Can you work these out from the model? Positions are in its coordinate system, mm. A direction names the side the tool comes from. Give positions to 0.01 mm unless a question says otherwise; leave off trailing zeros. Write each loop counter-clockwise with the first axis right and the second up, starting at its lowest first coordinate (ties: lowest second). Pieces come first, ordered by that corner, then holes.
from build123d import *

# Parameters (mm, degrees)
F1_DEPTH = 317.5
F4_DEPTH = 19.05
F5_DEPTH = 19.05


# Not quite as in the source:
# - a feature names something its author has since deleted; it is built from what else it names


with BuildPart() as f1:
    # F0 (on Front) → F1 (new body)
    with BuildSketch(Plane.XZ):
        with BuildLine():
            Line((152.4, 0), (0, 0))
            Line((0, 0), (0, -51.6636))
            Line((0, -51.6636), (8.7122, -51.6636))
            Line((8.7122, -51.6636), (8.7122, -18.1356))
            ThreePointArc((8.7122, -18.1356), (11.6879951031, -10.9513951031), (18.8722, -7.9756))
            Line((18.8722, -7.9756), (133.5278, -7.9756))
            ThreePointArc((133.5278, -7.9756), (140.7120048969, -10.9513951031), (143.6878, -18.1356))
            Line((143.6878, -18.1356), (143.6878, -51.6636))
            Line((143.6878, -51.6636), (152.4, -51.6636))
            Line((152.4, -51.6636), (152.4, 0))
        make_face()
    extrude(amount=F1_DEPTH)

    # F3 (on face) → F4 (join)
    with BuildSketch(Plane(origin=(0, 0, 0), x_dir=(-1, 0, 0), z_dir=(0, 1, 0))):
        with BuildLine():
            Line((-152.4, 108.3564), (-152.4, 0))
            Line((-152.4, 0), (0, 0))
            Line((0, 0), (0, 108.3564))
            ThreePointArc((0, 108.3564), (-1.4878975516, 111.9485024484), (-5.08, 113.4364))
            Line((-5.08, 113.4364), (-57.15, 113.4364))
            Line((-57.15, 113.4364), (-57.15, 81.6864))
            ThreePointArc((-57.15, 81.6864), (-76.2, 62.6364), (-95.25, 81.6864))
            Line((-95.25, 81.6864), (-95.25, 113.4364))
            Line((-95.25, 113.4364), (-147.32, 113.4364))
            ThreePointArc((-147.32, 113.4364), (-150.9121024484, 111.9485024484), (-152.4, 108.3564))
        make_face()
        with BuildLine():
            Line((-143.6878, -18.1356), (-143.6878, -51.6636))
            Line((-143.6878, -51.6636), (-8.7122, -51.6636))
            Line((-8.7122, -51.6636), (-8.7122, -18.1356))
            ThreePointArc((-8.7122, -18.1356), (-11.6879951031, -10.9513951031), (-18.8722, -7.9756))
            Line((-18.8722, -7.9756), (-133.5278, -7.9756))
            ThreePointArc((-133.5278, -7.9756), (-140.7120048969, -10.9513951031), (-143.6878, -18.1356))
        make_face()
        with BuildLine():
            Line((-152.4, 0), (-152.4, -51.6636))
            Line((-152.4, -51.6636), (-143.6878, -51.6636))
            Line((-143.6878, -51.6636), (-143.6878, -18.1356))
            ThreePointArc((-143.6878, -18.1356), (-140.7120048969, -10.9513951031), (-133.5278, -7.9756))
            Line((-133.5278, -7.9756), (-18.8722, -7.9756))
            ThreePointArc((-18.8722, -7.9756), (-11.6879951031, -10.9513951031), (-8.7122, -18.1356))
            Line((-8.7122, -18.1356), (-8.7122, -51.6636))
            Line((-8.7122, -51.6636), (0, -51.6636))
            Line((0, -51.6636), (0, 0))
            Line((0, 0), (-152.4, 0))
        make_face()
    extrude(amount=F4_DEPTH)

    # F2 (on face) → F5 (join)
    with BuildSketch(Plane.XZ.offset(317.5)):
        with BuildLine():
            Line((152.4, 0), (0, 0))
            Line((0, 0), (0, -100.33))
            ThreePointArc((0, -100.33), (2.2318463274, -105.7181536726), (7.62, -107.95))
            Line((7.62, -107.95), (144.78, -107.95))
            ThreePointArc((144.78, -107.95), (150.1681536726, -105.7181536726), (152.4, -100.33))
            Line((152.4, -100.33), (152.4, 0))
        make_face()
        with BuildLine():
            Line((28.5572737867, -76.085673397), (28.5940985013, -37.985673397))
            ThreePointArc((28.5940985013, -37.985673397), (38.2314841006, -28.6802259255), (47.6427262133, -38.214326603))
            Line((47.6427262133, -38.214326603), (47.6059014987, -76.314326603))
            ThreePointArc((47.6059014987, -76.314326603), (37.9659922536, -85.8300138104), (28.5572737867, -76.085673397))
        make_face(mode=Mode.SUBTRACT)
        with BuildLine():
            Line((104.7750042372, -76.2000004751), (104.7749957628, -38.099982679))
            ThreePointArc((104.7749957628, -38.099982679), (114.3000041857, -28.5750016435), (123.8249957628, -38.0999995249))
            Line((123.8249957628, -38.0999995249), (123.8250042372, -76.200017321))
            ThreePointArc((123.8250042372, -76.200017321), (114.2999958142, -85.7250194396), (104.7750042372, -76.2000004751))
        make_face(mode=Mode.SUBTRACT)
    extrude(amount=F5_DEPTH)


solid = f1.part
(1) Imagine slicing it at B-B, the plane y = -35. Write out the boundary of the cut face in (x, z), plus the area to 3 significant figures.
Returned:
outline: (0, -51.66) - (8.71, -51.66) - (8.71, -18.14) arc R10.16 cw to (18.87, -7.98) - (133.53, -7.98) arc R10.16 cw to (143.69, -18.14) - (143.69, -51.66) - (152.4, -51.66) - (152.4, 0) - (0, 0) - close
area: 2,020 mm2
(2) Imagine slicing it at D-D, the plane x = 76.2. Write out the boundary of the cut face in (y, z).
Returned:
outline: (-336.55, -107.95) - (-317.5, -107.95) - (-317.5, -7.98) - (0, -7.98) - (0, -51.66) - (19.05, -51.66) - (19.05, 62.64) - (0, 62.64) - (0, 0) - (-336.55, 0) - close
(3) Imagine slicing it at C-C, the plane x = 37.5. Write out the boundary of the cut face in (y, z).
Returned:
outline: (-336.55, -107.95) - (-317.5, -107.95) - (-317.5, -85.81) - (-336.55, -85.81) - close; (-336.55, -28.7) - (-317.5, -28.7) - (-317.5, -7.98) - (0, -7.98) - (0, -51.66) - (19.05, -51.66) - (19.05, 113.44) - (0, 113.44) - (0, 0) - (-336.55, 0) - close
(4) If I drill on L1, parallel to X at y = -44.5, z = -35; L2, parallel to Y at x = 57, z = -37; L3, parallel to Z at x = 101, y = -244.5, over which ranges is the centre line in solid material (lowest first)?
Returned:
L1: x = 0 to 8.71, 143.69 to 152.4
L2: y = -336.55 to -317.5, 0 to 19.05
L3: z = -7.98 to 0
(5) Will these pins go through, and if not, where does the flat tip stop? P1, Ø3, axis at x = 120, y = -32.5, coming from the +Z side; P2, Ø3, axis at x = 77, z = -75, coming from the +Y side.
Returned:
P1: stops at z = 0
P2: stops at y = -317.5
(6) If we mould it in two halves opening along Y, with no side actions, what happens to faces 6 (the face through (144, -113, -51.664)), 7 (the face through (77, 19.05, 32)), 8 (the face through (75, -317.5, -57))? For each: +Y half, -Y half, draft (parallel to the pull), parting line (faces both ways), or undercut.
Returned:
face 6: draft
face 7: +Y half
face 8: undercut
(7) Imagine slicing it at A-A, the plane z = -25. Write out the boundary of the cut face in (x, y).
Returned:
outline: (0, -336.55) - (152.4, -336.55) - (152.4, 19.05) - (0, 19.05) - close; hole (8.71, -317.5) - (143.69, -317.5) - (143.69, 0) - (8.71, 0) - close
(8) For faces 1 (the face through (140.63, -156.53, -10.87)), 2 (the face through (95.25, 9, 97)), 3 (the face through (77, -166, 0)), 4 (the face through (114.091, -326.892, -28.577)), 5 (the face through (114.509, -326.892, -85.723)), which set-ups out of +Z, -Z, +X, -X, +Y, -Y let a thin tool reach every point of the face, with its end or its side?
Returned:
face 1: -Z
face 2: +Z, +Y, -Y
face 3: +Z, +X, -X, -Y
face 4: -Y
face 5: +Y, -Y
